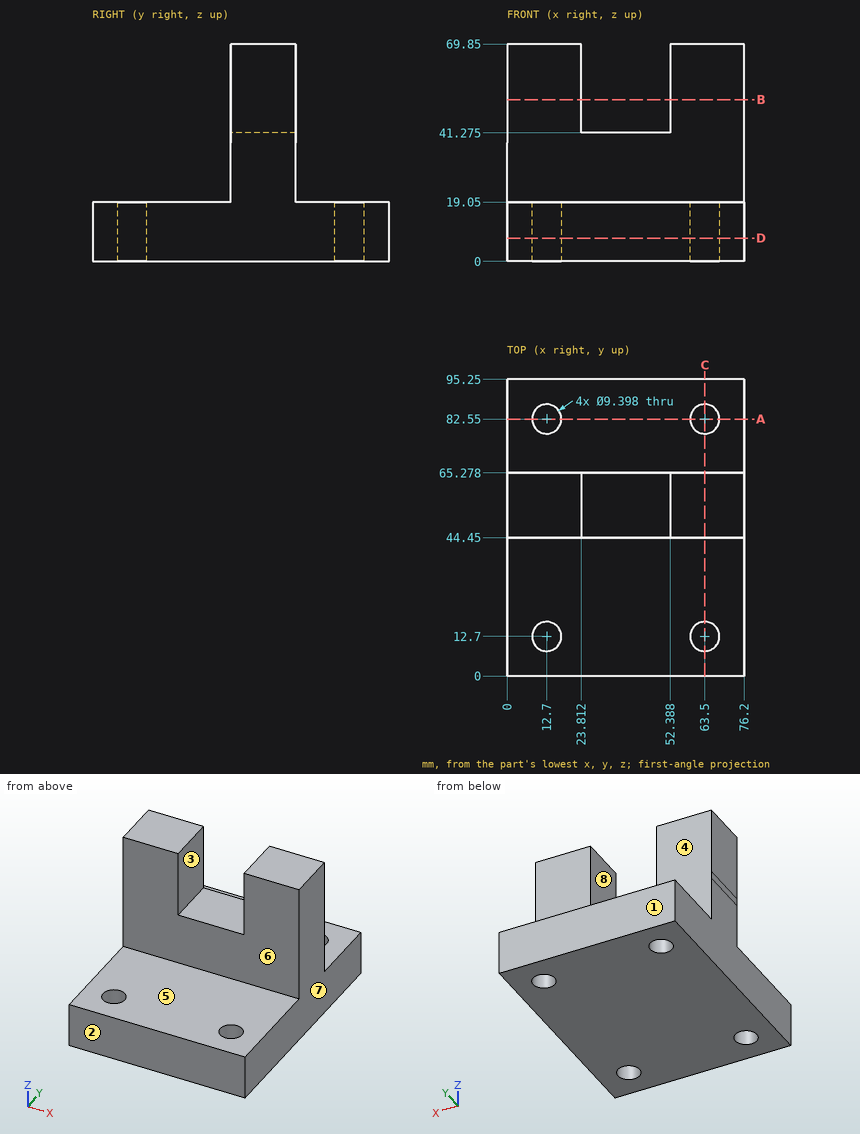
Geometry check sheet. Reference: drawing and pictorial views, mm from the part's lowest x, y, z. A direction names the side the tool comes from. Coordinates: 2 decimals unless noted, no trailing zeros. Write each loop counter-clockwise with the first axis right and the second up, starting at its lowest first coordinate (ties: lowest second). Pieces come first, ordered by that corner, then holes. Notation, with made-up numbers: (-15, 39.25) -> (13, 39.25) arc R21 cw to (13, 54.25) -> close; hole circle Ø11 at (87, 42.5). An arc over 180 degrees is marked (long way). One line per question, with ' | ' between items.
1. Draft check along X on the marked faces 6, 7 and 8. Enter one of: +X half, -X half, draft (parallel to the pull), parting line (faces both ways), or undercut.
Answers:
face 6: draft | face 7: +X half | face 8: undercut
2. Depth check by flat-ended pin: pin 1 Ø9 at (x, y) = (37.5, 77) entering from +Z; pin 2 Ø6 at (x, y) = (35.5, 54) entering from +Z (1 decimal); pin 3 Ø1.5 at (x, z) = (9.5, 30) entering from -Y. Enter the tip coordinate at first touch or a pass-through.
Answers:
pin 1: stops at z = 19.05 | pin 2: stops at z = 41.3 | pin 3: stops at y = 44.45
3. Cross-section at D-D on z = 7.5. Record the cut outline in (x, y), and give its area (3 significant figures).
Answers:
outline: (0, 0) -> (76.2, 0) -> (76.2, 95.25) -> (0, 95.25) -> close; hole circle Ø9.4 at (12.7, 12.7); hole circle Ø9.4 at (12.7, 82.55); hole circle Ø9.4 at (63.5, 12.7); hole circle Ø9.4 at (63.5, 82.55) | area: 6,980 mm²
4. Set-up check for the marked faces 1, 2, 3, 4 and 5: record each of +Z, -Z, +X, -X, +Y, -Y from which the full face is reachable in a straight line by a thin tool's end or side.
Answers:
face 1: +Z, -Z, +X, -X, +Y | face 2: +Z, -Z, +X, -X, -Y | face 3: +Z, +Y, -Y | face 4: +Z, +X, -X, +Y | face 5: +Z, +X, -X, -Y
5. Cross-section at A-A on y = 82.55. Record the cut outline in (x, z).
Answers:
outline: (0, 0) -> (8, 0) -> (8, 19.05) -> (0, 19.05) -> close; (17.4, 0) -> (58.8, 0) -> (58.8, 19.05) -> (17.4, 19.05) -> close; (68.2, 0) -> (76.2, 0) -> (76.2, 19.05) -> (68.2, 19.05) -> close
6. Cross-section at B-B on z = 52. Record the cut outline in (x, y).
Answers:
outline: (0, 44.45) -> (23.81, 44.45) -> (23.81, 65.28) -> (0, 65.28) -> close; (52.39, 44.45) -> (76.2, 44.45) -> (76.2, 65.28) -> (52.39, 65.28) -> close
7. Cross-section at C-C on x = 63.5. Record the cut outline in (y, z), and give its area (3 significant figures).
Answers:
outline: (0, 0) -> (8, 0) -> (8, 19.05) -> (0, 19.05) -> close; (17.4, 0) -> (77.85, 0) -> (77.85, 19.05) -> (65.28, 19.05) -> (65.28, 69.85) -> (44.45, 69.85) -> (44.45, 19.05) -> (17.4, 19.05) -> close; (87.25, 0) -> (95.25, 0) -> (95.25, 19.05) -> (87.25, 19.05) -> close | area: 2,510 mm²
8. Thickness scan on probe 1 along Y at (x, z) = (12.7, 7); probe 2 along X at (y, z) = (12, 9); probe 3 along X at (y, z) = (82, 10). Record the ranges inside material, lowest first. Write a range as from..to.
Answers:
probe 1: y = 0..8, 17.4..77.85, 87.25..95.25 | probe 2: x = 0..8.05, 17.35..58.85, 68.15..76.2 | probe 3: x = 0..8.03, 17.37..58.83, 68.17..76.2
